Geometry: final body of the model. Coordinates: model frame, mm. Give positions to 0.01 mm unless a question says otherwise; leave off trailing zeros. Loops run counter-clockwise (first coordinate to the right, second up) from the corner with the lowest first, then second, coordinate; pieces in that order, holes last. Notation, with made-up numbers: (82, -20.5) -> (125, -20.5) arc R10 ccw to (125, -9.5) -> close; hole circle Ø5 at (75.25, 64.25). An arc over 180 degrees is marked (long way). Answer in a Markdown table with one row per item. Add a question column.
1) First-contact query: P1, Ø6, axis at x = 187.32, z = 61.91, coming from the -Y side; P2, Ø8, axis at x = 0, z = 61.91, coming from the +Y side; P3, Ø11, axis at x = 187.32, z = -61.91, coming from the +Y side. Flat tips, straight axial feed; report the tip coordinate or a pass-through.
2) Section query A-A (y = 4.25). Return the cut outline in (x, z) (1 decimal).
3) Draft query along X for faces 1 (the flat face through (-3, 6.35, -1)), 2 (the conical face through (-171.814, 3.049, -62.377)). Return one class per face: +X half, -X half, draft (parallel to the pull), parting line (faces both ways), or undercut.
4) Line query: line 1 (X direction, y = 1, z = -62); line 2 (Z direction, x = 2, y = 0.75); line 3 (Z direction, x = -168.5, y = 1). Output: solid intervals per line, ascending. Write a range as from..to.
```python
from build123d import *

# Parameters (mm, degrees)
SKETCH1_W                                     = 431.8
SKETCH1_H                                     = 152.4
BOSS_EXTRUDE1_DEPTH                           = 6.35
CHAMFER1_SIZE                                 = 6.35
CSK_FOR_1_4_FLAT_HEAD_MACHINE_SCREW1_AT_COUNT = 2
CSK_FOR_1_4_FLAT_HEAD_MACHINE_SCREW1_AT_PITCH = 187.325
CSK_FOR_1_4_FLAT_HEAD_MACHINE_SCREW1_2_COUNT  = 2
CSK_FOR_1_4_FLAT_HEAD_MACHINE_SCREW1_2_PITCH  = 355.6
CSK_FOR_1_4_FLAT_HEAD_MACHINE_SCREW1_3_COUNT  = 2
CSK_FOR_1_4_FLAT_HEAD_MACHINE_SCREW1_3_PITCH  = 376.542149865
CSK_FOR_1_4_FLAT_HEAD_MACHINE_SCREW1_4_COUNT  = 2
CSK_FOR_1_4_FLAT_HEAD_MACHINE_SCREW1_4_PITCH  = 123.825
CSK_FOR_1_4_FLAT_HEAD_MACHINE_SCREW1_5_COUNT  = 2
CSK_FOR_1_4_FLAT_HEAD_MACHINE_SCREW1_5_PITCH  = 224.551299818


with BuildPart() as part:
    # Sketch1 → Boss-Extrude1 (new body)
    with BuildSketch(Plane(origin=(0, 0, 0), x_dir=(1, 0, 0), z_dir=(0, 1, 0))):
        Rectangle(SKETCH1_W, SKETCH1_H)
    extrude(amount=BOSS_EXTRUDE1_DEPTH)

    # Chamfer1
    chamfer1_edges = [part.edges().sort_by_distance(p)[0] for p in [
        (0, 6.35, 76.2),
        (0, 6.35, -76.2),
    ]]
    chamfer(chamfer1_edges, length=CHAMFER1_SIZE - 0.0001)  # a hair under: the kernel refuses the full size

    # Sketch3 → CSK for 1/4 Flat Head Machine Screw1 (revolve, cut)
    with BuildSketch(Plane(origin=(187.325, 6.35, 61.9125), x_dir=(0, 0, 1), z_dir=(1, 0, 0))):
        Polygon((0, 0), (0, 6.35), (3.3782, 6.35), (3.3782, 3.520932584), (6.4389, 0), align=None)
    csk_for_1_4_flat_head_machine_screw1 = revolve(axis=Axis((187.325, 12.7, 61.9125), (0, -1, 0)), mode=Mode.SUBTRACT)

    # CSK for 1/4 Flat Head Machine Screw1 at: CSK for 1/4 Flat Head Machine Screw1 ×2
    with Locations(*[(-i * CSK_FOR_1_4_FLAT_HEAD_MACHINE_SCREW1_AT_PITCH, 0, 0) for i in range(1, CSK_FOR_1_4_FLAT_HEAD_MACHINE_SCREW1_AT_COUNT)]):
        add(csk_for_1_4_flat_head_machine_screw1, mode=Mode.SUBTRACT)

    # CSK for 1_4 Flat Head Machine Screw1 2: CSK for 1/4 Flat Head Machine Screw1 ×2
    with Locations(*[(-i * CSK_FOR_1_4_FLAT_HEAD_MACHINE_SCREW1_2_PITCH, 0, 0) for i in range(1, CSK_FOR_1_4_FLAT_HEAD_MACHINE_SCREW1_2_COUNT)]):
        add(csk_for_1_4_flat_head_machine_screw1, mode=Mode.SUBTRACT)

    # CSK for 1_4 Flat Head Machine Screw1 3: CSK for 1/4 Flat Head Machine Screw1 ×2
    with Locations(*[Vector(-0.9443829864131722, 0, -0.32884764705458697) * (i * CSK_FOR_1_4_FLAT_HEAD_MACHINE_SCREW1_3_PITCH) for i in range(1, CSK_FOR_1_4_FLAT_HEAD_MACHINE_SCREW1_3_COUNT)]):
        add(csk_for_1_4_flat_head_machine_screw1, mode=Mode.SUBTRACT)

    # CSK for 1_4 Flat Head Machine Screw1 4: CSK for 1/4 Flat Head Machine Screw1 ×2
    with Locations(*[(0, 0, -i * CSK_FOR_1_4_FLAT_HEAD_MACHINE_SCREW1_4_PITCH) for i in range(1, CSK_FOR_1_4_FLAT_HEAD_MACHINE_SCREW1_4_COUNT)]):
        add(csk_for_1_4_flat_head_machine_screw1, mode=Mode.SUBTRACT)

    # CSK for 1_4 Flat Head Machine Screw1 5: CSK for 1/4 Flat Head Machine Screw1 ×2
    with Locations(*[Vector(-0.8342191746462441, 0, -0.5514330137492126) * (i * CSK_FOR_1_4_FLAT_HEAD_MACHINE_SCREW1_5_PITCH) for i in range(1, CSK_FOR_1_4_FLAT_HEAD_MACHINE_SCREW1_5_COUNT)]):
        add(csk_for_1_4_flat_head_machine_screw1, mode=Mode.SUBTRACT)


solid = part.part
```
Evaluation:
| question | item | result |
|---|---|---|
| 1 | P1 | through |
| 1 | P2 | y = 3.55 |
| 1 | P3 | y = 5.28 |
| 2 | outline | (-215.9, -72) -> (215.9, -72) -> (215.9, 72) -> (-215.9, 72) -> close; hole circle Ø9.2 at (-168.3, -61.9); hole circle Ø9.2 at (-168.3, 61.9); hole circle Ø9.2 at (0, -61.9); hole circle Ø9.2 at (0, 61.9); hole circle Ø9.2 at (187.3, -61.9); hole circle Ø9.2 at (187.3, 61.9) |
| 3 | face 1 | draft |
| 3 | face 2 | undercut |
| 4 | line 1 | -215.9..-171.65, -164.9..-3.38, 3.38..183.95, 190.7..215.9 |
| 4 | line 2 | -75.45..-64.64, -59.19..59.19, 64.64..75.45 |
| 4 | line 3 | -75.2..-65.28, -58.54..58.54, 65.28..75.2 |
